Geometry: final body of the model. Coordinates: model frame, mm. A direction names the side the tool comes from. Give positions to 0.01 mm unless a question says otherwise; leave off trailing zeros. Write each loop counter-clockwise with the first axis right and the second up, starting at its lowest first coordinate (ties: lowest second). Pieces come first, ordered by that corner, then holes.
Q1. Pin query (flat end, axial travel): pin 1 (3 mm diameter, centred on x = 143, y = 69.5, fed in from +Z). Return the tip coordinate at first contact, or that it passes through.
Q2. Cut plane C-C on x = 20. Return the cut outline in (y, z).
Q3. Line query: L1, parallel to Y at x = 81.9, z = 12.65; L2, parallel to Y at x = 219.5, z = 12.45; L3, parallel to Y at x = 161.5, z = 15. Output: solid intervals per line, ascending.
Q4. Cut plane D-D on y = 53.5. Count the separate pieces of the cut face and the enclosed holes in it, plus the area to 3 significant figures.
Q5. Cut plane B-B on z = 3.5. Return the cut outline in (x, y), plus the area to 3 significant figures.
Q6. Reachability of faces 5 (the face through (153.1, 20.48, 13.01)), 6 (the face through (144.51, 6.95, 18.88)), 7 (the face through (144, 0, 9)) from +Z, -Z, +X, -X, +Y, -Y: full face, straight path, thin tool, end or side. Return the list, or none.
Q7. Draft query along X for faces 1 (the face through (-2, 51, 9)), 2 (the face through (145.8, 100.4, 20)), 3 (the face through (264, 20.48, 13.01)), 4 (the face through (144, -2, 9)). Return one class per face: pulls with the +X half, pulls with the -X half, needs draft (parallel to the pull), parting line crosses it, or undercut.
```python
from build123d import *

# Parameters (mm, degrees)
SKETCH_W        = 293
SKETCH_H        = 103
PAD_DEPTH       = 20
SKETCH001_W     = 277
SKETCH001_H     = 87
POCKET_DEPTH    = 8
CHAMFER_SIZE    = 5
FILLET_R        = 1
THICKNESS_T     = 2
SKETCH003_W     = 103
SKETCH003_H     = 35
SKETCH003_W_2   = 20
POCKET002_DEPTH = 5
SKETCH004_R     = 3.25
POCKET003_DEPTH = 2


with BuildPart() as part:
    # Sketch → Pad (new body)
    with BuildSketch(Plane.XY):
        with Locations((146.5, 51.5)):
            Rectangle(SKETCH_W, SKETCH_H)
    extrude(amount=PAD_DEPTH)

    # Sketch001 (on Face6 of Pad) → Pocket (cut)
    with BuildSketch(Plane.XY.offset(20)):
        with Locations((146.5, 51.5)):
            Rectangle(SKETCH001_W, SKETCH001_H)
    extrude(amount=-POCKET_DEPTH, mode=Mode.SUBTRACT)

    # Chamfer
    chamfer_edges = [part.edges().sort_by_distance(p)[0] for p in [
        (8, 51.5, 20),
        (146.5, 95, 20),
        (146.5, 8, 20),
        (285, 51.5, 20),
    ]]
    chamfer(chamfer_edges, length=CHAMFER_SIZE)

    # Fillet
    fillet_edges = [part.edges().sort_by_distance(p)[0] for p in [
        (146.5, 0, 20),
        (0, 51.5, 20),
        (146.5, 103, 20),
        (293, 51.5, 20),
    ]]
    fillet(fillet_edges, radius=FILLET_R)

    # Thickness
    thickness_openings = [part.faces().sort_by_distance(p)[0] for p in [
        (146.5, 51.5, 0),
    ]]
    offset(amount=THICKNESS_T, openings=thickness_openings)

    # Sketch003 → Pocket002 (cut)
    with BuildSketch(Plane.XY.offset(14)):
        with Locations((76.5, 64)):
            Rectangle(SKETCH003_W, SKETCH003_H)
        with Locations((172, 64)):
            Rectangle(SKETCH003_W_2, SKETCH003_H)
        with Locations((255.1, 64)):
            Rectangle(SKETCH003_W_2, SKETCH003_H)
    extrude(amount=-POCKET002_DEPTH, mode=Mode.SUBTRACT)

    # Sketch004 (on Face48 of Pocket002) → Pocket003 (cut)
    with BuildSketch(Plane.XY.offset(14)):
        with Locations((26.7, 19.5)):
            Circle(SKETCH004_R)
        with Locations((40.5, 19.5)):
            Circle(SKETCH004_R)
        with Locations((54.3, 19.5)):
            Circle(SKETCH004_R)
        with Locations((68.1, 19.5)):
            Circle(SKETCH004_R)
        with Locations((81.9, 19.5)):
            Circle(SKETCH004_R)
        with Locations((95.7, 19.5)):
            Circle(SKETCH004_R)
        with Locations((109.5, 19.5)):
            Circle(SKETCH004_R)
        with Locations((123.3, 19.5)):
            Circle(SKETCH004_R)
        with Locations((150, 19.5)):
            Circle(SKETCH004_R)
        with Locations((163.8, 19.5)):
            Circle(SKETCH004_R)
        with Locations((177.6, 19.5)):
            Circle(SKETCH004_R)
        with Locations((191.4, 19.5)):
            Circle(SKETCH004_R)
        with Locations((219.5, 19.5)):
            Circle(SKETCH004_R)
        with Locations((233.3, 19.5)):
            Circle(SKETCH004_R)
        with Locations((247.1, 19.5)):
            Circle(SKETCH004_R)
        with Locations((260.9, 19.5)):
            Circle(SKETCH004_R)
    extrude(amount=-POCKET003_DEPTH, mode=Mode.SUBTRACT)


solid = part.part
```
Data:
1. pin 1: stops at z = 14
2. outline: (-2, 0) - (0, 0) - (0, 19) arc R1 cw to (1, 20) - (3, 20) - (8, 15) - (8, 12) - (95, 12) - (95, 15) - (100, 20) - (102, 20) arc R1 cw to (103, 19) - (103, 0) - (105, 0) - (105, 19) arc R3 ccw to (102, 22) - (100, 22) arc R2 ccw to (98.59, 21.41) - (93.59, 16.41) arc R2 ccw to (93, 15) - (93, 14) - (10, 14) - (10, 15) arc R2 ccw to (9.41, 16.41) - (4.41, 21.41) arc R2 ccw to (3, 22) - (1, 22) arc R3 ccw to (-2, 19) - close
3. L1: y = -2 to 0, 8 to 16.25, 22.75 to 46.5, 81.5 to 95, 103 to 105
3. L2: y = -2 to 0, 8 to 16.25, 22.75 to 95, 103 to 105
3. L3: y = -2 to 0, 8 to 10, 93 to 95, 103 to 105
4. separate pieces: 4
4. enclosed holes: 0
4. area: 403 mm2
5. outline: (-2, 0) arc R2 ccw to (0, -2) - (293, -2) arc R2 ccw to (295, 0) - (295, 103) arc R2 ccw to (293, 105) - (0, 105) arc R2 ccw to (-2, 103) - close; hole (0, 0) - (293, 0) - (293, 103) - (0, 103) - close
5. area: 1,600 mm2
6. face 5: +Z, -Z
6. face 6: +Z
6. face 7: -Z
7. face 1: pulls with the -X half
7. face 2: undercut
7. face 3: undercut
7. face 4: needs draft
